Geometry: final body of the model. Coordinates: model frame, mm. A direction names the side the tool comes from. Coordinates: 2 decimals unless noted, no trailing zeros. Loops run counter-clockwise (first coordinate to the right, second up) from the corner with the lowest first, then second, coordinate; pieces in that order, holes last. Notation, with made-up numbers: (-2.5, -12.75) -> (6.5, -12.75) arc R18 cw to (6.5, 2.25) -> close; hole circle Ø4 at (67.25, -2). An arc over 180 degrees is marked (long way). One line per item, written item: value. Start each with the question number.
Item 1: Section query A-A on x = 0. Return loops of the section in (y, z).
Item 2: Section query C-C on y = -6. Return loops of the section in (x, z).
Item 3: Contact query for flat-ended pins moving along their axis: pin 1 Ø1.5 at (y, z) = (-12, 3.5) entering from -X; pin 2 Ø5 at (y, z) = (-8, -8) entering from -X. Output: stop coordinate, or through.
Item 4: Set-up query: faces 4 (the flat face through (0, -15, 0)), 5 (the cylindrical face through (5.96, -14.01, 1.88)), 6 (the flat face through (0, -4, 0)). Return all of +Z, -Z, +X, -X, +Y, -Y with unobstructed straight access to the full face (end or side cutting, diameter ignored); none if empty.
Item 5: Ray query, probe 1 along Z at (x, y) = (0, -2.95); probe 2 along Z at (x, y) = (0, -13.75); probe 3 along X at (y, z) = (-3.25, -1). Return the intervals inside material, ascending. Write a range as from..to.
Item 6: Section query B-B on z = 0. Return loops of the section in (x, y).
Item 7: Mould query, pull axis X, two halves, no side actions, for faces 1 (the flat face through (2, 0, -2)), 2 (the cylindrical face through (0, -2, -2)), 3 (the cylindrical face through (-2.17, -6.42, -9.76)). Classes: +X half, -X half, draft (parallel to the pull), parting line (faces both ways), or undercut.
Item 8: Section query D-D on y = -1.75. Return loops of the section in (x, z).
from build123d import *

# Parameters (mm, degrees)
F0_R     = 10
F1_DEPTH = 15
F2_R     = 3
F3_R     = 1
F4_R     = 2
F5_DEPTH = 4
F6_R     = 7
F6_R_2   = 6.25
F8_DEPTH = 2


with BuildPart() as f1:
    # F0 (on Front) → F1 (new body)
    with BuildSketch(Plane.XZ):
        Circle(F0_R)
    extrude(amount=F1_DEPTH)

    # F2
    f2_edges = [f1.edges().sort_by_distance(p)[0] for p in [
        (-10, -15, 0),
    ]]
    fillet(f2_edges, radius=F2_R)

    # F3
    f3_edges = [f1.edges().sort_by_distance(p)[0] for p in [
        (-10, 0, 0),
    ]]
    fillet(f3_edges, radius=F3_R)

    # F4 (on face) → F5 (cut)
    with BuildSketch(Plane(origin=(0, 0, 0), x_dir=(-1, 0, 0), z_dir=(0, 1, 0))):
        Circle(F4_R)
    extrude(amount=-F5_DEPTH, mode=Mode.SUBTRACT)

    # F6 (on face) → F8 (cut)
    with BuildSketch(Plane.XZ.offset(15)):
        Circle(F6_R)
        Circle(F6_R_2, mode=Mode.SUBTRACT)
    extrude(amount=-F8_DEPTH, mode=Mode.SUBTRACT)


solid = f1.part
Reply:
1. outline: (-15, -7) arc R3 ccw to (-12, -10) -> (-1, -10) arc R1 ccw to (0, -9) -> (0, -2) -> (-4, -2) -> (-4, 2) -> (0, 2) -> (0, 9) arc R1 ccw to (-1, 10) -> (-12, 10) arc R3 ccw to (-15, 7) -> (-13, 7) -> (-13, 6.25) -> (-15, 6.25) -> (-15, -6.25) -> (-13, -6.25) -> (-13, -7) -> close
2. outline: circle Ø20 at (0, 0)
3. pin 1: stops at x = -9.61
3. pin 2: stops at x = -8.35
4. face 4: +Z, -Z, +X, -X, -Y
4. face 5: -Y
4. face 6: +Y
5. probe 1: z = -10..-2, 2..10
5. probe 2: z = -9.44..-7, -6.25..6.25, 7..9.44
5. probe 3: x = -9.95..-1.73, 1.73..9.95
6. outline: (-10, -12) arc R3 ccw to (-7, -15) -> (-7, -13) -> (-6.25, -13) -> (-6.25, -15) -> (6.25, -15) -> (6.25, -13) -> (7, -13) -> (7, -15) arc R3 ccw to (10, -12) -> (10, -1) arc R1 ccw to (9, 0) -> (2, 0) -> (2, -4) -> (-2, -4) -> (-2, 0) -> (-9, 0) arc R1 ccw to (-10, -1) -> close
7. face 1: draft
7. face 2: undercut
7. face 3: parting line
8. outline: circle Ø20 at (0, 0); hole circle Ø4 at (0, 0)
